Design review of the part built by this model. Coordinates are the model's own, in mm. Face numbers are marked on the shaded views. A direction names the side the tool comes from. Give positions to 0.01 mm unless a question says otherwise; leave off trailing zeros. Loops run counter-clockwise (first coordinate to the right, second up) from the corner with the lowest first, then second, coordinate; pieces in that order, holes last. Notation, with made-up numbers: M -6.75,-36.5 L -0.75,-36.5 A36 ccw -0.75,1.5 Z; hole C -24.5,6 d1. An arc over 180 degrees is marked long. Use CSV: the item, a comma, the result in double quotes.
from build123d import *

# Parameters (mm, degrees)
SKETCH1_W           = 210
SKETCH1_H           = 170
BOSS_EXTRUDE1_DEPTH = 7
SKETCH2_W           = 180
SKETCH2_H           = 135
BOSS_EXTRUDE2_DEPTH = 60


with BuildPart() as part:
    # Sketch1 → Boss-Extrude1 (new body)
    with BuildSketch(Plane(origin=(0, 0, 0), x_dir=(1, 0, 0), z_dir=(0, 1, 0))):
        with Locations((105, 85)):
            Rectangle(SKETCH1_W, SKETCH1_H)
    extrude(amount=BOSS_EXTRUDE1_DEPTH)

    # Sketch2 → Boss-Extrude2 (add)
    with BuildSketch(Plane(origin=(0, 7, 0), x_dir=(1, 0, 0), z_dir=(0, 1, 0))):
        Polygon((210, 170), (0, 170), (0, 160), (10, 160), (10, 25), (10, 20.500436989), (10, 15), (204, 15), (204, 18.199432026), (204, 25), (204, 160), (210, 160), align=None)
        with Locations((107, 92.5)):
            Rectangle(SKETCH2_W, SKETCH2_H, mode=Mode.SUBTRACT)
    extrude(amount=BOSS_EXTRUDE2_DEPTH)


solid = part.part
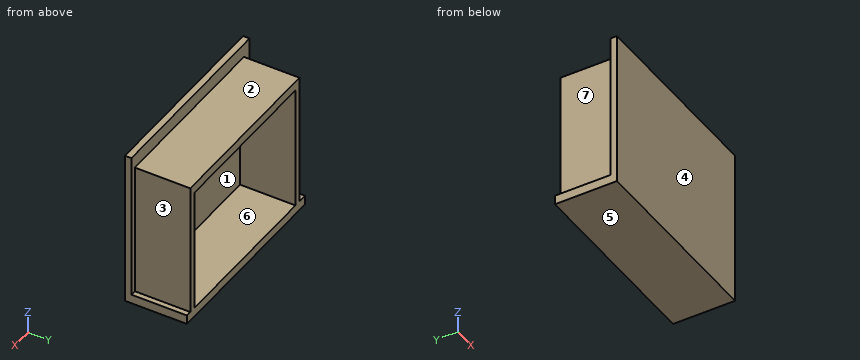
(1) Clearance check with flat-ended pins moving along their axes: P1, Ø18, axis at y = 29.5, z = -110, coming from the +X side; P2, Ø3, axis at x = 5, y = 42.5, coming from the +Z side; P3, Ø3, axis at x = 177.5, y = 21, coming from the +Z side; P4, Ø6, axis at x = 61.5, z = -109, coming from the -Y side. State where each tip first meets the part, or that it passes through.
A:
P1,"x = 204"
P2,"z = -160"
P3,"z = -15"
P4,"y = 0"
(2) We need section B-B on y = 28.5. State the section outline as (x, z) points, then the cut area to 3 significant figures.
A:
outline,"M 0,-170 L 210,-170 L 210,-160 L 204,-160 L 204,-15 L 10,-15 L 10,-160 L 0,-160 Z; hole M 17,-160 L 197,-160 L 197,-25 L 17,-25 Z"
area,"5,930 mm²"
(3) The part is to be moulded in two halves that separate along Z. For the marked faces 5, 6 and 7, say which applies: released by +Z, released by -Z, zero draft, split by the parting line, or undercut.
A:
face 5,"released by -Z"
face 6,"undercut"
face 7,"zero draft"
(4) We need section A-A on z = -108. State the section outline as (x, y) points, then the cut area to 3 significant figures.
A:
outline,"M 0,0 L 210,0 L 210,7 L 204,7 L 204,67 L 197,67 L 197,7 L 17,7 L 17,67 L 10,67 L 10,7 L 0,7 Z"
area,"2,310 mm²"
(5) Wall thickness on line 1 along X through (y, z) = (47, -135); line 2 along Z through (x, y) = (167, 48.5); line 3 along Z through (x, y) = (14, 31): over which ranges is each line inside the solid? List them lowest first. Write a range as [from, to].
A:
line 1,"[10, 17], [197, 204]"
line 2,"[-170, -160], [-25, -15]"
line 3,"[-170, -15]"
(6) Machinability: for the marked faces 1, 2, 3 and 4, which of the approach directions +Z, -Z, +X, -X, +Y, -Y give a long, thin tool a straight path to every point of the face, cutting with its end or side? Answer none if there is none.
A:
face 1,"+Y"
face 2,"+Z, +X, -X, +Y"
face 3,"+Z, +X, +Y"
face 4,"+Z, -Z, +X, -X, -Y"
(7) We need section C-C on x = 186.5. State the section outline as (y, z) points, then the cut area to 3 significant figures.
A:
outline,"M 0,-170 L 67,-170 L 67,-160 L 7,-160 L 7,-25 L 67,-25 L 67,-15 L 7,-15 L 7,0 L 0,0 Z"
area,"2,390 mm²"
